Work out the finished part from the listing and answer in its coordinate system (mm). A direction names the side the tool comes from. Round coordinates to 2 decimals unless told otherwise and drop trailing zeros. Loops run counter-clockwise (first coordinate to the right, second up) from the corner with the lowest first, then second, coordinate; pieces in that order, holes last. Notation, with made-up numbers: (45.5, -5.5) - (55.5, -5.5) arc R14 cw to (55.5, 3.5) - close; hole circle Ø6 at (75.5, 7). An arc over 180 degrees is marked (long way). Return JSON: item names as keys, results as strings.
from build123d import *

# Parameters (mm, degrees)
BOSS_EXTRUDE1_DEPTH       = 8
BOSS_EXTRUDE1_DEPTH_BACK  = 8
SKETCH1_W                 = 40
SKETCH1_H                 = 16
SHELL1_T                  = -2
SKETCH3_R                 = 4.470610275
CUT_EXTRUDE1_DEPTH        = 10
SKETCH4_W                 = 12
SKETCH4_H                 = 14
SKETCH4_R                 = 2.75
BOSS_EXTRUDE2_DEPTH       = 2.4
LPATTERN1_COUNT           = 2
LPATTERN1_PITCH           = 7.4
LPATTERN2_COUNT           = 2
LPATTERN2_PITCH           = 16
LPATTERN2_COPY_1_SKETCH_W = 12
LPATTERN2_COPY_1_SKETCH_H = 14
LPATTERN2_COPY_1_SKETCH_R = 2.75
LPATTERN2_COPY_1_DEPTH    = 2.4
BOSS_EXTRUDE4_DEPTH       = 5
LPATTERN3_COUNT           = 2
LPATTERN3_PITCH           = 16
BOSS_EXTRUDE6_START       = -16
BOSS_EXTRUDE6_DEPTH       = 16
SKETCH12_R                = 5.25
CUT_EXTRUDE3_DEPTH        = 45.824637279
LPATTERN4_COUNT           = 2
LPATTERN4_PITCH           = 36
BOSS_EXTRUDE5_DEPTH       = 2.4


with BuildPart() as part:
    # Sketch1 → Boss-Extrude1 (new, two sides: drawn at the far end of the back side and taken through both)
    with BuildSketch(Plane.XY.offset(-BOSS_EXTRUDE1_DEPTH_BACK)):
        with Locations((3, 0)):
            Rectangle(SKETCH1_W, SKETCH1_H)
    extrude(amount=BOSS_EXTRUDE1_DEPTH + BOSS_EXTRUDE1_DEPTH_BACK)

    # Shell1
    shell1_openings = [part.faces().sort_by_distance(p)[0] for p in [
        (3, 8, 0),
    ]]
    offset(amount=SHELL1_T, openings=shell1_openings, kind=Kind.INTERSECTION)

    # Sketch3 → Cut-Extrude1 (cut)
    with BuildSketch(Plane.ZY.offset(17)):
        Circle(SKETCH3_R)
    extrude(amount=-CUT_EXTRUDE1_DEPTH, mode=Mode.SUBTRACT)

    # Sketch4 → Boss-Extrude2 (add)
    with BuildSketch(Plane(origin=(-7, 0, 0), x_dir=(0, 0, -1), z_dir=(1, 0, 0))):
        with Locations((0, 1)):
            Rectangle(SKETCH4_W, SKETCH4_H)
        Circle(SKETCH4_R, mode=Mode.SUBTRACT)
    boss_extrude2 = extrude(amount=BOSS_EXTRUDE2_DEPTH)

    # LPattern1: Boss-Extrude2 ×2
    with Locations(*[(i * LPATTERN1_PITCH, 0, 0) for i in range(1, LPATTERN1_COUNT)]):
        add(boss_extrude2)

    # LPattern2: Boss-Extrude2 ×2
    with Locations(*[(i * LPATTERN2_PITCH, 0, 0) for i in range(1, LPATTERN2_COUNT)]):
        add(boss_extrude2)

    # LPattern2 copy 1 sketch → LPattern2 copy 1 (add)
    with BuildSketch(Plane(origin=(16.4, 0, 0), x_dir=(0, 0, -1), z_dir=(1, 0, 0))):
        with Locations((0, 1)):
            Rectangle(LPATTERN2_COPY_1_SKETCH_W, LPATTERN2_COPY_1_SKETCH_H)
        Circle(LPATTERN2_COPY_1_SKETCH_R, mode=Mode.SUBTRACT)
    extrude(amount=LPATTERN2_COPY_1_DEPTH)

    # Sketch6 → Boss-Extrude4 (add)
    with BuildSketch(Plane.ZY.offset(-16.4)):
        Polygon((-4.25, 2.453738644), (-4.25, 8), (-6, 8), (-6, -6), (6, -6), (6, 8), (4.25, 8), (4.25, 2.453738644), (4.25, -2.453738644), (0, -4.907477288), (-4.25, -2.453738644), align=None)
    boss_extrude4 = extrude(amount=BOSS_EXTRUDE4_DEPTH)

    # LPattern3: Boss-Extrude4 ×2
    with Locations(*[(-i * LPATTERN3_PITCH, 0, 0) for i in range(1, LPATTERN3_COUNT)]):
        add(boss_extrude4)

    # Sketch11 → Boss-Extrude6 (add)
    with BuildSketch(Plane.XZ.offset(8).offset(BOSS_EXTRUDE6_START)):
        with BuildLine():
            ThreePointArc((-10.251996289, 32.330297023), (-14.636700237, 20.445466564), (-17, 8))
            Line((-17, 8), (-14.58633595, 8))
            ThreePointArc((-14.58633595, 8), (-12.290169012, 19.925625473), (-8.0768576, 31.316013195))
            Line((-8.0768576, 31.316013195), (-10.251996289, 32.330297023))
        make_face()
        with BuildLine():
            ThreePointArc((-17, 8), (-17.41945058, 0), (-17, -8))
            Line((-17, -8), (-17, 8))
        make_face()
        with BuildLine():
            Line((-17, 8), (-17, -8))
            Line((-17, -8), (-14.58633595, -8))
            ThreePointArc((-14.58633595, -8), (-15.01945058, 0), (-14.58633595, 8))
            Line((-14.58633595, 8), (-17, 8))
        make_face()
        with BuildLine():
            ThreePointArc((-17, -8), (-14.636700237, -20.445466564), (-10.251996289, -32.330297023))
            Line((-10.251996289, -32.330297023), (-8.0768576, -31.316013195))
            ThreePointArc((-8.0768576, -31.316013195), (-12.290169012, -19.925625473), (-14.58633595, -8))
            Line((-14.58633595, -8), (-17, -8))
        make_face()
    extrude(amount=BOSS_EXTRUDE6_DEPTH)

    # Sketch12 → Cut-Extrude3 (cut, through all)
    with BuildSketch(Plane.ZY.offset(7)):
        with Locations(Location((0, 0, 0), (0, 0, 108.866979722))):
            Circle(SKETCH12_R)
    extrude(amount=CUT_EXTRUDE3_DEPTH, mode=Mode.SUBTRACT)


with BuildPart() as lpattern4_1:
    # LPattern4: pattern copy
    add(part.part.moved(Location(Vector(0, 0, -1) * (1 * LPATTERN4_PITCH))))


with BuildPart() as part_1:
    add(part.part)

    add(lpattern4_1.part)  # Boss-Extrude5 merges LPattern4_1
    # Sketch8 → Boss-Extrude5 (add)
    with BuildSketch(Plane(origin=(23, 0, 0), x_dir=(0, 0, -1), z_dir=(1, 0, 0))):
        Polygon((47, -15), (-11, -15), (-17, -9), (-17, 9), (-11, 15), (47, 15), (53, 9), (53, -9), align=None)
    extrude(amount=-BOSS_EXTRUDE5_DEPTH)


solid = part_1.part
1) Section B-B (z = -19) is taken. Give the vertices of the cut face in (x, y).
Verdict:
{"outline": "(-15.51, -8) - (-12.54, -8) - (-12.54, 8) - (-15.51, 8) - close; (20.6, -15) - (23, -15) - (23, 15) - (20.6, 15) - close"}
2) Find the intervals of material crossed by L1, parallel to Z at x = -1.5, y = -2.25; L2, parallel to Z at x = 5.5, y = -5.75; L3, parallel to Y at x = -5, z = -36, in increasing order.
Verdict:
{"L1": "z = -44 to -40.25, -31.75 to -28, -8 to -4.25, 4.25 to 8", "L2": "z = -44 to -42, -30 to -28, -8 to -6, 6 to 8", "L3": "y = -8 to -2.75, 2.75 to 8"}
3) Flat-ended cylindrical pins translate along their axes: pin 1 (7 mm diameter, centred on x = 7, y = 1, fed in from -Z); pin 2 (13 mm diameter, centred on x = 1, y = 1, fed in from +Z); pin 3 (4 mm diameter, centred on x = -2.5, z = -3.5, fed in from +Y); pin 4 (4 mm diameter, centred on x = -11, y = -10.5, fed in from -Z). Find the tip coordinate at first contact, or state that the pin passes through.
Verdict:
{"pin 1": "stops at z = -44", "pin 2": "stops at z = 8", "pin 3": "stops at y = 8", "pin 4": "passes through"}
4) Section A-A (x = 14) is taken. Give the vertices of the cut face in (y, z).
Verdict:
{"outline": "(-8, -44) - (8, -44) - (8, -40.25) - (-2.45, -40.25) - (-4.91, -36) - (-2.45, -31.75) - (8, -31.75) - (8, -28) - (-8, -28) - close; (-8, -8) - (8, -8) - (8, -4.25) - (-2.45, -4.25) - (-4.91, 0) - (-2.45, 4.25) - (8, 4.25) - (8, 8) - (-8, 8) - close"}
5) Section C-C (y = 0) is taken. Count the separate pieces of the cut face and the enclosed holes in it, and give its area (3 significant figures).
Verdict:
{"separate pieces": "1", "enclosed holes": "3", "area": "887 mm2"}
6) Determine the mould class of faces 1 (the cylindrical face through (10.183, -2.685, 0.596)), 2 (the cylindrical face through (-13.023, 0.112, -10.44)) for opening direction X: pulls with the +X half, pulls with the -X half, needs draft (parallel to the pull), parting line crosses it, or undercut.
Verdict:
{"face 1": "needs draft", "face 2": "undercut"}
7) Section D-D (y = -10.25) is taken. Give the vertices of the cut face in (x, z), and give its area (3 significant figures).
Verdict:
{"outline": "(20.6, -51.75) - (23, -51.75) - (23, 15.75) - (20.6, 15.75) - close", "area": "162 mm2"}
8) A tool of negligible diameter and unlimited length cuts with its end or side. For faces 3 (the flat face through (1, 8, -6)), 4 (the flat face through (-4.6, 3, -36)), 5 (the cylindrical face through (10.183, 0.121, -33.253)), from which of +Z, -Z, +X, -X, +Y, -Y can it reach the whole face along a straight path? Write none if from no direction.
Verdict:
{"face 3": "+Z, -Z, -X, +Y", "face 4": "+Y", "face 5": "-X"}
